The model under review builds one solid part; all positions refer to its coordinate system, in mm. Face numbers are marked on the shaded views. A direction names the side the tool comes from. Coordinates: 2 decimals unless noted, no trailing zeros. Write each loop counter-clockwise with the first axis right and the second up, starting at its lowest first coordinate (ties: lowest second). Pieces come first, ordered by that corner, then holes.
1) Add section C-C, the plane x = 9.5. State the section outline as (y, z) points.
2) Add section A-A, the plane z = 0. State the section outline as (x, y) points (3 decimals).
3) For line 1 (Y direction, x = -19.5, z = -24); line 2 (X direction, y = 112.25, z = 0) (3 decimals); line 3 (X direction, y = 67, z = 30), list the stretches that pass through material, from the lowest coordinate up.
4) Add section D-D, the plane x = 18. State the section outline as (y, z) points, then the cut area to 3 significant figures.
5) Add section B-B, the plane y = 22. State the section outline as (x, z) points.
6) Mouldability with a two-part tool opening along X and no side actions: class the marked faces 1, 2 and 3 as released by +X, released by -X, zero draft, split by the parting line, or undercut.
7) Machinability: for the marked faces 4 and 5, which of the approach directions +Z, -Z, +X, -X, +Y, -Y give a long, thin tool a straight path to every point of the face, cutting with its end or side? Answer none if there is none.
8) For P1, Ø8, axis at x = 16, z = -6.5, coming from the +Y side; P2, Ø6, axis at y = 126, z = 17.5, coming from the +X side; P3, Ø5, axis at x = 1.5, z = -25, coming from the +Y side, all flat-tipped, find the tip position at first contact; note any pin that passes through.
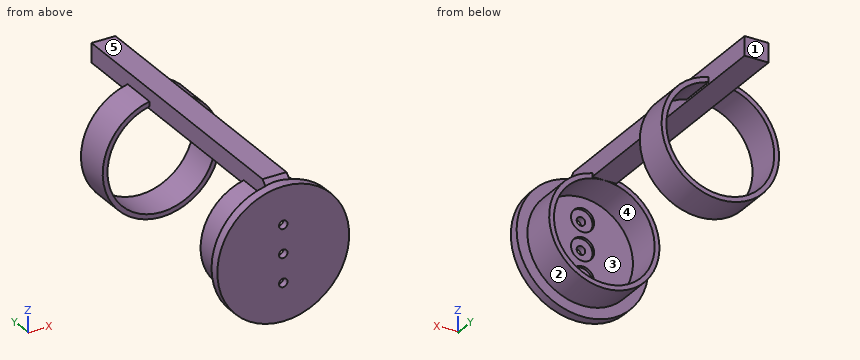
from build123d import *

# Parameters (mm, degrees)
SKETCH1_R                 = 34.925
BOSS_EXTRUDE1_DEPTH       = 5.08
SKETCH3_W                 = 12.7
SKETCH3_H                 = 10.16
BOSS_EXTRUDE2_DEPTH       = 152.4
SKETCH4_R                 = 29.21
SKETCH4_R_2               = 26.67
EXTRUDE_THIN1_DEPTH       = 19.05
ADVANCEDHOLE3_START       = 3.65
ADVANCEDHOLE3_OUTLINE_R   = 6.12
ADVANCEDHOLE3_DEPTH       = 1.43
ADVANCEDHOLE3_2_OUTLINE_R = 2.25
ADVANCEDHOLE3_2_DEPTH     = 3.65
CHAMFER1_SIZE             = 2.54
SKETCH14_R                = 31.115
SKETCH14_R_2              = 28.575
EXTRUDE_THIN3_DEPTH       = 19.05


# Read off the part's stored shape, not the designer's step: AdvancedHole3
with BuildPart() as part:
    # Sketch1 → Boss-Extrude1 (new body)
    with BuildSketch(Plane(origin=(0, 0, 0), x_dir=(1, 0, 0), z_dir=(0, 1, 0))):
        with Locations(Location((0, 0, 0), (0, 0, 270))):
            Circle(SKETCH1_R)
    extrude(amount=BOSS_EXTRUDE1_DEPTH)

    # Sketch3 → Boss-Extrude2 (add)
    with BuildSketch(Plane(origin=(0, 5.08, 0), x_dir=(1, 0, 0), z_dir=(0, 1, 0))):
        with Locations((0, -31.75)):
            Rectangle(SKETCH3_W, SKETCH3_H)
    extrude(amount=BOSS_EXTRUDE2_DEPTH)

    # Sketch4 → Extrude-Thin1 (add)
    with BuildSketch(Plane(origin=(0, 5.08, 0), x_dir=(1, 0, 0), z_dir=(0, 1, 0))):
        Circle(SKETCH4_R)
        Circle(SKETCH4_R_2, mode=Mode.SUBTRACT)
    extrude(amount=EXTRUDE_THIN1_DEPTH)

    # AdvancedHole3 outline → AdvancedHole3 (cut)
    with BuildSketch(Plane(origin=(0, 0, 0), x_dir=(1, 0, 0), z_dir=(0, 1, 0)).offset(ADVANCEDHOLE3_START)):
        with Locations((0, 15)):
            Circle(ADVANCEDHOLE3_OUTLINE_R)
        with Locations((0, -15)):
            Circle(ADVANCEDHOLE3_OUTLINE_R)
        Circle(ADVANCEDHOLE3_OUTLINE_R)
    extrude(amount=ADVANCEDHOLE3_DEPTH, mode=Mode.SUBTRACT)

    # AdvancedHole3 2 outline → AdvancedHole3 2 (cut)
    with BuildSketch(Plane(origin=(0, 0, 0), x_dir=(1, 0, 0), z_dir=(0, 1, 0))):
        with Locations((0, 15)):
            Circle(ADVANCEDHOLE3_2_OUTLINE_R)
        with Locations((0, -15)):
            Circle(ADVANCEDHOLE3_2_OUTLINE_R)
        Circle(ADVANCEDHOLE3_2_OUTLINE_R)
    extrude(amount=ADVANCEDHOLE3_2_DEPTH, mode=Mode.SUBTRACT)

    # Chamfer1
    # the kernel refuses this chamfer: 2.54 mm, written as the material it takes off along each edge
    with BuildSketch(Plane(origin=(12.882074789, 5.08, 36.83), x_dir=(0, -0.02749587661058625, -0.9996219169112968), z_dir=(-1, 0, 0))) as chamfer1_piece_1_section:
        Polygon((CHAMFER1_SIZE * 0.999621916911, -CHAMFER1_SIZE * 0.0274958766106), (-CHAMFER1_SIZE * 0.0274958766106, -CHAMFER1_SIZE * 0.999621916911), (0, 0), align=None)
    chamfer1_piece_1 = extrude(amount=25.764149579, mode=Mode.PRIVATE)
    chamfer1_piece_1 = chamfer1_piece_1 - Plane(origin=(0, 5.934504944, 0), x_dir=(0, 0, 1), z_dir=(0, -1, 0)) * Cylinder(34.925, 62, mode=Mode.PRIVATE)
    add(chamfer1_piece_1, mode=Mode.SUBTRACT)

    # Sketch14 → Extrude-Thin3 (add)
    with BuildSketch(Plane.ZX.offset(106.68)):
        Circle(SKETCH14_R)
        Circle(SKETCH14_R_2, mode=Mode.SUBTRACT)
    extrude(amount=EXTRUDE_THIN3_DEPTH)


solid = part.part
Geometry results:
1. outline: (0, -33.61) - (5.08, -33.61) - (5.08, -27.62) - (24.13, -27.62) - (24.13, -24.92) - (5.08, -24.92) - (5.08, 24.92) - (24.13, 24.92) - (24.13, 27.62) - (5.08, 27.62) - (5.08, 33.61) - (0, 33.61) - close; (106.68, -29.63) - (125.73, -29.63) - (125.73, -26.95) - (106.68, -26.95) - close; (106.68, 26.95) - (125.73, 26.95) - (125.73, 29.63) - (106.68, 29.63) - close
2. outline: (-34.925, 0) - (-2.25, 0) - (-2.25, 3.65) - (-6.12, 3.65) - (-6.12, 5.08) - (-26.67, 5.08) - (-26.67, 24.13) - (-29.21, 24.13) - (-29.21, 5.08) - (-34.925, 5.08) - close; (-31.115, 106.68) - (-28.575, 106.68) - (-28.575, 125.73) - (-31.115, 125.73) - close; (2.25, 0) - (34.925, 0) - (34.925, 5.08) - (29.21, 5.08) - (29.21, 24.13) - (26.67, 24.13) - (26.67, 5.08) - (6.12, 5.08) - (6.12, 3.65) - (2.25, 3.65) - close; (28.575, 106.68) - (31.115, 106.68) - (31.115, 125.73) - (28.575, 125.73) - close
3. line 1: y = 0 to 5.08, 106.68 to 125.73
3. line 2: x = -31.115 to -28.575, 28.575 to 31.115
3. line 3: x = -6.35 to 6.35
4. outline: (0, -29.93) - (5.08, -29.93) - (5.08, -23) - (24.13, -23) - (24.13, -19.68) - (5.08, -19.68) - (5.08, 19.68) - (24.13, 19.68) - (24.13, 23) - (5.08, 23) - (5.08, 29.93) - (0, 29.93) - close; (106.68, -25.38) - (125.73, -25.38) - (125.73, -22.19) - (106.68, -22.19) - close; (106.68, 22.19) - (125.73, 22.19) - (125.73, 25.38) - (106.68, 25.38) - close
4. area: 552 mm2
5. outline: (-6.35, 28.51) arc R29.21 ccw (long way) to (6.35, 28.51) - (6.35, 36.83) - (-6.35, 36.83) - close; hole circle Ø53.34 at (0, 0)
6. face 1: zero draft
6. face 2: split by the parting line
6. face 3: undercut
7. face 4: +Y
7. face 5: +Z, +X, -X, +Y, -Y
8. P1: stops at y = 5.08
8. P2: stops at x = 27.52
8. P3: stops at y = 24.13
